For this review, take the finished solid that the model builds, in its own axes (mm). Face numbers are marked on the shaded views. A direction names the side the tool comes from. Coordinates: 2 decimals unless noted, no trailing zeros. Order: outer loops, then holes, each group sorted by start corner. A loop starts at its lowest first (then second) coordinate and runs counter-clockwise, first axis right, second up. Notation, with made-up numbers: (63.25, -10) -> (112.25, -10) arc R20 cw to (112.25, 19) -> close; hole circle Ø11 at (25, -15). An arc over 180 degrees is marked (long way). Answer as a JSON object with one key per item and string values. Group by question number.
1) Wall thickness on L1, parallel to X at y = 1, z = 2.5; L2, parallel to Y at x = 15, z = 5.25; L3, parallel to Z at x = -16, y = 17.5: over which ranges is each line inside the solid? List them lowest first.
2) Add section A-A, the plane z = 6.75. Write out the cut boundary in (x, y).
3) Machinability: for the marked faces 1 and 2, which of the approach directions +Z, -Z, +X, -X, +Y, -Y give a long, thin tool a straight path to every point of the face, cutting with its end or side? Answer none if there is none.
4) Add section C-C, the plane x = 32.5. Write out the cut boundary in (y, z).
5) Add section D-D, the plane z = 13.5. Write out the cut boundary in (x, y), then the cut area to 3 significant figures.
6) Draft analysis for pull direction Y (two halves, no side actions). For the marked faces 3, 4, 5 and 6, state which applies: +Y half, -Y half, draft (parallel to the pull), parting line (faces both ways), or undercut.
7) Add section B-B, the plane y = -2.5. Write out the cut boundary in (x, z), then the cut area to 3 significant figures.
from build123d import *

# Parameters (mm, degrees)
SKETCH_W        = 84
SKETCH_H        = 59
PAD_DEPTH       = 20
SKETCH002_W     = 80
SKETCH002_H     = 55
POCKET_DEPTH    = 18
SKETCH003_W     = 5
SKETCH003_H     = 2
PAD001_DEPTH    = 1
SKETCH004_W     = 5
SKETCH004_H     = 2
PAD002_DEPTH    = 1
POCKET001_DEPTH = 2
FILLET_R        = 0.5
FILLET001_R     = 0.4
FILLET002_R     = 0.5
FILLET003_R     = 0.5


with BuildPart() as part:
    # Sketch → Pad (new body)
    with BuildSketch(Plane.XY):
        with Locations((3, 0)):
            Rectangle(SKETCH_W, SKETCH_H)
    extrude(amount=PAD_DEPTH)

    # Sketch002 (on Face5 of Pad) → Pocket (cut)
    with BuildSketch(Plane(origin=(0, 0, 0), x_dir=(1, 0, 0), z_dir=(0, 0, -1))):
        with Locations((3, 0)):
            Rectangle(SKETCH002_W, SKETCH002_H)
    extrude(amount=-POCKET_DEPTH, mode=Mode.SUBTRACT)

    # Sketch003 (on Face8 of Pocket) → Pad001 (join)
    with BuildSketch(Plane.XZ.offset(-27.5)):
        with Locations((-18.5, 3)):
            Rectangle(SKETCH003_W, SKETCH003_H)
        with Locations((18.5, 3)):
            Rectangle(SKETCH003_W, SKETCH003_H)
    extrude(amount=PAD001_DEPTH)

    # Sketch004 (on Face10 of Pad001) → Pad002 (join)
    with BuildSketch(Plane(origin=(0, -27.5, 0), x_dir=(-1, 0, 0), z_dir=(0, 1, 0))):
        with Locations((-18.5, 3)):
            Rectangle(SKETCH004_W, SKETCH004_H)
        with Locations((18.5, 3)):
            Rectangle(SKETCH004_W, SKETCH004_H)
    extrude(amount=PAD002_DEPTH)

    # Sketch005 (on Face3 of Pad002) → Pocket001 (cut)
    with BuildSketch(Plane.YZ.offset(45)):
        with BuildLine():
            ThreePointArc((-21.5, 0), (-18, -3.5), (-14.5, 0))
            Line((-14.5, 0), (-14.5, 8.5))
            ThreePointArc((-14.5, 8.5), (-18, 12), (-21.5, 8.5))
            Line((-21.5, 0), (-21.5, 8.5))
        make_face()
        with BuildLine():
            ThreePointArc((-5, 0), (-2.5, -2.5), (0, 0))
            Line((0, 0), (0, 8.5))
            ThreePointArc((0, 8.5), (-2.5, 11), (-5, 8.5))
            Line((-5, 0), (-5, 8.5))
        make_face()
        with BuildLine():
            ThreePointArc((3, 0), (5.5, -2.5), (8, 0))
            Line((8, 0), (8, 8.5))
            ThreePointArc((8, 8.5), (5.5, 11), (3, 8.5))
            Line((3, 0), (3, 8.5))
        make_face()
        with BuildLine():
            ThreePointArc((11, 0), (13.5, -2.5), (16, 0))
            Line((16, 0), (16, 8.5))
            ThreePointArc((16, 8.5), (13.5, 11), (11, 8.5))
            Line((11, 0), (11, 8.5))
        make_face()
    extrude(amount=-POCKET001_DEPTH, mode=Mode.SUBTRACT)

    # Fillet
    fillet_edges = [part.edges().sort_by_distance(p)[0] for p in [
        (3, 29.5, 20),
        (-39, 0, 20),
        (3, -29.5, 20),
        (45, 0, 20),
    ]]
    fillet(fillet_edges, radius=FILLET_R)

    # Fillet001
    fillet001_edges = [part.edges().sort_by_distance(p)[0] for p in [
        (45, 29.5, 9.75),
        (45, -29.5, 9.75),
        (-39, 29.5, 9.75),
        (-39, -29.5, 9.75),
    ]]
    fillet(fillet001_edges, radius=FILLET001_R)

    # Fillet002
    fillet002_edges = [part.edges().sort_by_distance(p)[0] for p in [
        (-18.5, -26.5, 2),
        (-21, -26.5, 3),
        (-18.5, -26.5, 4),
        (-16, -26.5, 3),
        (16, -26.5, 3),
        (18.5, -26.5, 2),
        (21, -26.5, 3),
        (18.5, -26.5, 4),
    ]]
    fillet(fillet002_edges, radius=FILLET002_R)

    # Fillet003
    fillet003_edges = [part.edges().sort_by_distance(p)[0] for p in [
        (-21, 26.5, 3),
        (-18.5, 26.5, 4),
        (-18.5, 26.5, 2),
        (-16, 26.5, 3),
        (18.5, 26.5, 2),
        (16, 26.5, 3),
        (18.5, 26.5, 4),
        (21, 26.5, 3),
    ]]
    fillet(fillet003_edges, radius=FILLET003_R)


solid = part.part
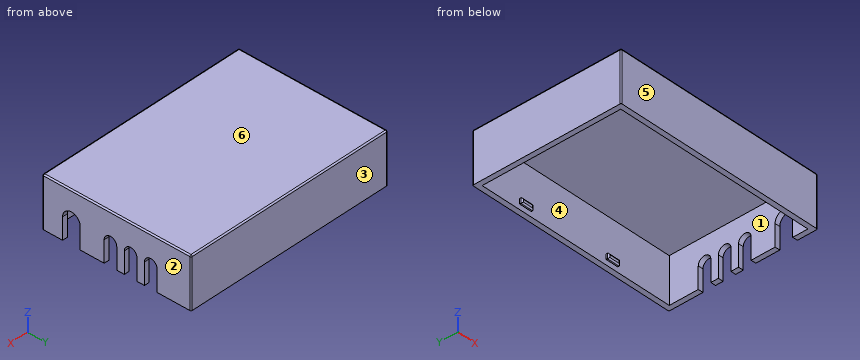
Output values:
{
 "1": {"L1": "x = -39 to -37, 43 to 45", "L2": "y = -29.5 to -27.5, 27.5 to 29.5", "L3": "z = 18 to 20"},
 "2": {"outline": "(-39, -29.1) arc R0.4 ccw to (-38.6, -29.5) -> (44.6, -29.5) arc R0.4 ccw to (45, -29.1) -> (45, -21.5) -> (43, -21.5) -> (43, -27.5) -> (-37, -27.5) -> (-37, 27.5) -> (43, 27.5) -> (43, 16) -> (45, 16) -> (45, 29.1) arc R0.4 ccw to (44.6, 29.5) -> (-38.6, 29.5) arc R0.4 ccw to (-39, 29.1) -> close; (43, -14.5) -> (45, -14.5) -> (45, -5) -> (43, -5) -> close; (43, 0) -> (45, 0) -> (45, 3) -> (43, 3) -> close; (43, 8) -> (45, 8) -> (45, 11) -> (43, 11) -> close"},
 "3": {"face 1": "-Z", "face 2": "+Z, -Z, +X, +Y, -Y"},
 "4": {"outline": "(-29.5, 0) -> (-27.5, 0) -> (-27.5, 18) -> (27.5, 18) -> (27.5, 0) -> (29.5, 0) -> (29.5, 19.5) arc R0.5 ccw to (29, 20) -> (-29, 20) arc R0.5 ccw to (-29.5, 19.5) -> close"},
 "5": {"outline": "(-39, -29.1) arc R0.4 ccw to (-38.6, -29.5) -> (44.6, -29.5) arc R0.4 ccw to (45, -29.1) -> (45, 29.1) arc R0.4 ccw to (44.6, 29.5) -> (-38.6, 29.5) arc R0.4 ccw to (-39, 29.1) -> close; hole (-37, -27.5) -> (43, -27.5) -> (43, 27.5) -> (-37, 27.5) -> close", "area": "556 mm²"},
 "6": {"face 3": "+Y half", "face 4": "undercut", "face 5": "-Y half", "face 6": "draft"},
 "7": {"outline": "(-39, 0) -> (-37, 0) -> (-37, 18) -> (43, 18) -> (43, 11) -> (45, 11) -> (45, 19.5) arc R0.5 ccw to (44.5, 20) -> (-38.5, 20) arc R0.5 ccw to (-39, 19.5) -> close", "area": "218 mm²"}
}
